from build123d import *

# Parameters (mm, degrees)
SKETCH1_W             = 160
SKETCH1_H             = 140
BOSS_EXTRUDE1_DEPTH   = 2
F_3_0MM_DOWEL_HOLE1_D = 3
F_1_5MM_DOWEL_HOLE4_D = 18
F_3_0MM_DOWEL_HOLE2_D = 7
FILLET2_R             = 2
SKETCH22_W            = 16
SKETCH22_H            = 8
CUT_EXTRUDE1_DEPTH    = 2


with BuildPart() as part:
    # Sketch1 → Boss-Extrude1 (new body)
    with BuildSketch(Plane(origin=(0, 0, 0), x_dir=(1, 0, 0), z_dir=(0, 1, 0))):
        Rectangle(SKETCH1_W, SKETCH1_H)
    extrude(amount=BOSS_EXTRUDE1_DEPTH)

    # Ø3.0mm Dowel Hole1 (through all)
    with Locations(Plane(origin=(0, 2, 0), x_dir=(1, 0, 0), z_dir=(0, 1, 0))):
        with Locations((-76, 66), (76, 66), (76, -66), (-76, -66)):
            Hole(F_3_0MM_DOWEL_HOLE1_D / 2)

    # Ø1.5mm Dowel Hole4 (through all)
    with Locations(Plane(origin=(0, 2, 0), x_dir=(1, 0, 0), z_dir=(0, 1, 0))):
        with Locations((56.336, -6.348), (-9.958, -28.878)):
            Hole(F_1_5MM_DOWEL_HOLE4_D / 2)

    # Ø3.0mm Dowel Hole2 (through all)
    with Locations(Plane(origin=(0, 2, 0), x_dir=(1, 0, 0), z_dir=(0, 1, 0))):
        with Locations((-9.958, 40), (25.042, 40), (-9.958, 15), (25.042, 15), (25.042, -28.878)):
            Hole(F_3_0MM_DOWEL_HOLE2_D / 2)

    # Fillet2
    fillet2_edges = [part.edges().sort_by_distance(p)[0] for p in [
        (80, 2, 0),
        (0, 2, -70),
        (-80, 2, 0),
        (0, 2, 70),
    ]]
    fillet(fillet2_edges, radius=FILLET2_R - 0.0001)  # a hair under: the kernel refuses the full size

    # Sketch22 → Cut-Extrude1 (cut)
    with BuildSketch(Plane(origin=(0, 2, 0), x_dir=(1, 0, 0), z_dir=(0, 1, 0))):
        with Locations((60, -51)):
            Rectangle(SKETCH22_W, SKETCH22_H)
    extrude(amount=-CUT_EXTRUDE1_DEPTH, mode=Mode.SUBTRACT)


solid = part.part
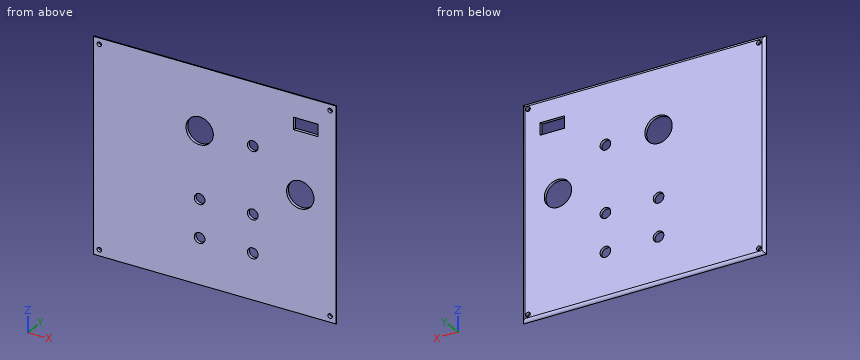
Verification items for the finished model (mm, model axes). Round coordinates to 2 decimals unless told otherwise and drop trailing zeros.
(1) Material ranges on line 1 (X direction, y = 1.1, z = 66); line 2 (X direction, y = 1.65, z = -66); line 3 (Z direction, x = 64.5, y = 1.45), recorded low to high.
Returned:
line 1: x = -79.67 to -77.5, -74.5 to 74.5, 77.5 to 79.67
line 2: x = -79.13 to -77.5, -74.5 to 74.5, 77.5 to 79.13
line 3: z = -69.38 to 2.56, 10.14 to 47, 55 to 69.38
(2) Depth check by flat-ended pin: pin 1 Ø1.5 at (x, z) = (-43.5, 2) entering from -Y; pin 2 Ø6.5 at (x, z) = (-9.958, -15) entering from +Y; pin 3 Ø0.6 at (y, z) = (1, 50.5) entering from +X; pin 4 Ø0.6 at (y, z) = (1.5, 52.5) entering from -X. Enter the tip coordinate at first touch or a pass-through.
Returned:
pin 1: stops at y = 0
pin 2: passes through
pin 3: stops at x = 79.87
pin 4: stops at x = -79.6
(3) Section check A-A (z = -15). Give the number of separate pieces and of enclosed holes in the cut face, plus the area to 3 significant figures.
Returned:
separate pieces: 3
enclosed holes: 0
area: 290 mm2
